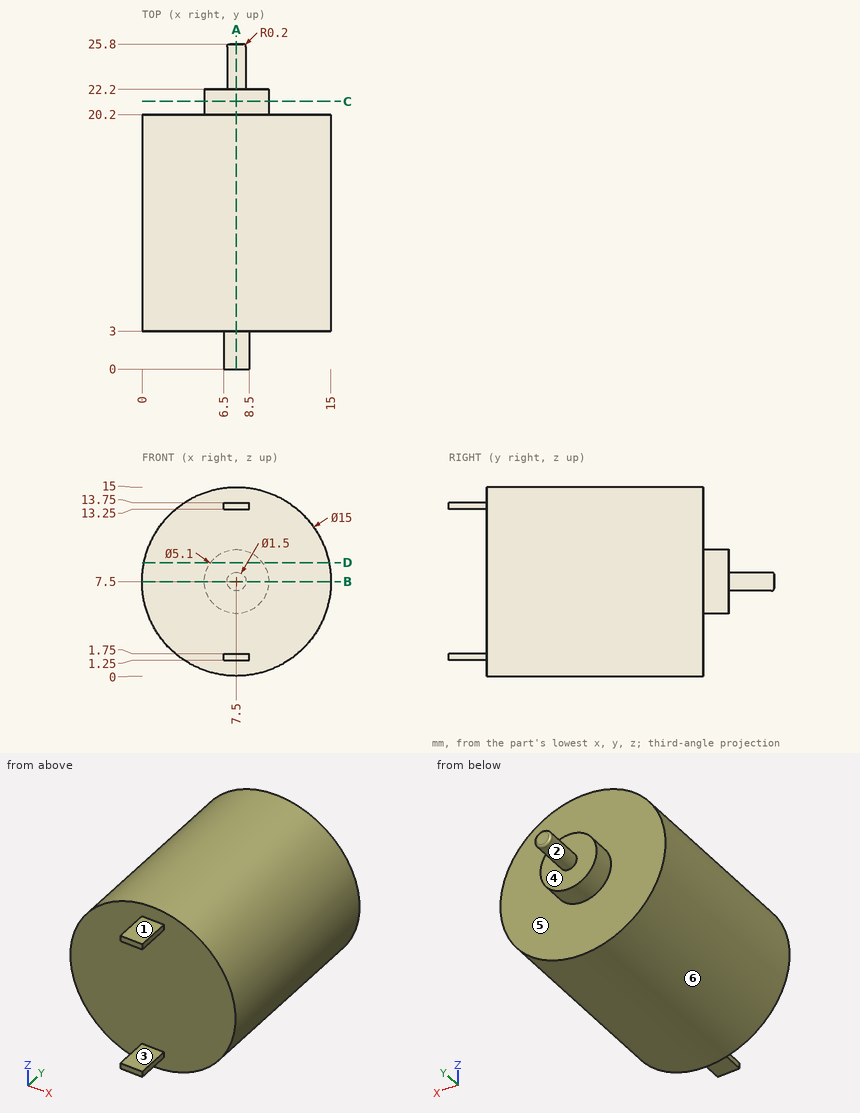
Geometry check sheet. Reference: drawing and pictorial views, mm from the part's lowest x, y, z. A direction names the side the tool comes from. Coordinates: 2 decimals unless noted, no trailing zeros. Loops run counter-clockwise (first coordinate to the right, second up) from the corner with the lowest first, then second, coordinate; pieces in that order, holes last. Notation, with made-up numbers: (80, -11.75) - (125, -11.75) arc R29 ccw to (125, 22.25) - close; hole circle Ø6 at (9.5, -24.5). An arc over 180 degrees is marked (long way). Return JSON: item names as keys, results as strings.
1. Section check C-C, the plane y = 21.25. Record the boundary of the cut face in (x, z).
Established:
{"outline": "circle Ø5.1 at (7.5, 7.5)"}
2. Tool access check on the marked faces 5 and 6. Record the directions out of +Z, -Z, +X, -X, +Y, -Y that give a thin tool (end or side, any length) a straight path to the whole face; none if there is none.
Established:
{"face 5": "+Y", "face 6": "+Y, -Y"}
3. Thickness scan on L1, parallel to Y at x = 10.75, z = 5.25; L2, parallel to Y at x = 8.5, z = 6; L3, parallel to X at y = 4.5, z = 7.75. Record the ranges inside material, lowest first.
Established:
{"L1": "y = 3 to 20.2", "L2": "y = 3 to 22.2", "L3": "x = 0 to 15"}
4. Section check A-A, the plane x = 7.5. Record the boundary of the cut face in (y, z), then the cut area to 3 significant figures.
Established:
{"outline": "(0, 1.25) - (3, 1.25) - (3, 0) - (20.2, 0) - (20.2, 4.95) - (22.2, 4.95) - (22.2, 6.75) - (25.6, 6.75) arc R0.2 ccw to (25.8, 6.95) - (25.8, 8.05) arc R0.2 ccw to (25.6, 8.25) - (22.2, 8.25) - (22.2, 10.05) - (20.2, 10.05) - (20.2, 15) - (3, 15) - (3, 13.75) - (0, 13.75) - (0, 13.25) - (3, 13.25) - (3, 1.75) - (0, 1.75) - close", "area": "277 mm2"}
5. Mould release check, pull along Z, two halves, no side actions. Record for the marked faces 1, 2, 3 and 4: +Z half, -Z half, draft (parallel to the pull), parting line (faces both ways), or undercut.
Established:
{"face 1": "+Z half", "face 2": "parting line", "face 3": "undercut", "face 4": "draft"}
6. Section check D-D, the plane z = 9. Record the boundary of the cut face in (x, y), then the cut area to 3 significant figures.
Established:
{"outline": "(0.15, 3) - (14.85, 3) - (14.85, 20.2) - (9.56, 20.2) - (9.56, 22.2) - (5.44, 22.2) - (5.44, 20.2) - (0.15, 20.2) - close", "area": "261 mm2"}
7. Section check B-B, the plane z = 7.5. Record the boundary of the cut face in (x, y).
Established:
{"outline": "(0, 3) - (15, 3) - (15, 20.2) - (10.05, 20.2) - (10.05, 22.2) - (8.25, 22.2) - (8.25, 25.6) arc R0.2 ccw to (8.05, 25.8) - (6.95, 25.8) arc R0.2 ccw to (6.75, 25.6) - (6.75, 22.2) - (4.95, 22.2) - (4.95, 20.2) - (0, 20.2) - close"}
8. Go/stop test with flat-tipped pins: pin 1 (1.6 mm diameter, centred on x = 7.5, y = 1, fed in from -Z); pin 2 (6 mm diameter, centred on x = 6, z = 11, fed in from +Y); pin 3 (6 mm diameter, centred on x = 2.5, y = 10, fed in from +Z). Record where each tip stops, or that it passes through.
Established:
{"pin 1": "stops at z = 1.25", "pin 2": "stops at y = 22.2", "pin 3": "stops at z = 14.73"}
